Here's how the part is built. I have some questions about the finished solid (model axes, mm). A direction names the side the tool comes from. Give positions to 0.01 mm unless a question says otherwise; leave off trailing zeros. Order: outer loops, then holes, each group sorted by start corner. A loop starts at its lowest first (then second) coordinate and runs counter-clockwise, first axis right, second up.
from build123d import *

# Parameters (mm, degrees)
SKETCH1_R           = 1.5
BOSS_EXTRUDE1_DEPTH = 3
CUT_EXTRUDE1_DEPTH  = 4


with BuildPart() as part:
    # Sketch1 → Boss-Extrude1 (new body)
    with BuildSketch(Plane.XY):
        with BuildLine():
            Line((-36.448598131, -26.168224299), (-36.448598131, -23.168224299))
            Line((-36.448598131, -23.168224299), (-34.837367865, 22.971373688))
            ThreePointArc((-34.837367865, 22.971373688), (-33.618438039, 25.709134902), (-30.839804557, 26.831775701))
            Line((-30.839804557, 26.831775701), (-19.702559656, 26.831775701))
            ThreePointArc((-19.702559656, 26.831775701), (-17.165801235, 25.924485955), (-15.779830266, 23.614204058))
            Line((-15.779830266, 23.614204058), (-6.448598131, -23.168224299))
            Line((-6.448598131, -23.168224299), (-6.448598131, -26.168224299))
            Line((-6.448598131, -26.168224299), (-16.448598131, -26.168224299))
            Line((-16.448598131, -26.168224299), (-16.448598131, -23.168224299))
            Line((-16.448598131, -23.168224299), (-26.448598131, -23.168224299))
            Line((-26.448598131, -23.168224299), (-26.448598131, -26.168224299))
            Line((-26.448598131, -26.168224299), (-36.448598131, -26.168224299))
        make_face()
        with Locations((-21.448598131, 18.831775701)):
            Circle(SKETCH1_R, mode=Mode.SUBTRACT)
        with BuildLine():
            Line((-27.448598131, 4.074261176), (-27.448598131, 0.074261176))
            ThreePointArc((-27.448598131, 0.074261176), (-28.948598131, -1.425738824), (-30.448598131, 0.074261176))
            Line((-30.448598131, 0.074261176), (-30.448598131, 4.074261176))
            ThreePointArc((-30.448598131, 4.074261176), (-28.948598131, 5.574261176), (-27.448598131, 4.074261176))
        make_face(mode=Mode.SUBTRACT)
        with BuildLine():
            Line((-19.448598131, 4.074261176), (-19.448598131, 0.074261176))
            ThreePointArc((-19.448598131, 0.074261176), (-20.948598131, -1.425738824), (-22.448598131, 0.074261176))
            Line((-22.448598131, 0.074261176), (-22.448598131, 4.074261176))
            ThreePointArc((-22.448598131, 4.074261176), (-20.948598131, 5.574261176), (-19.448598131, 4.074261176))
        make_face(mode=Mode.SUBTRACT)
        with BuildLine():
            ThreePointArc((-28.948598131, 18.831775701), (-26.75189899, 13.528474842), (-21.448598131, 11.331775701))
            ThreePointArc((-21.448598131, 11.331775701), (-19.948598131, 12.831775701), (-21.448598131, 14.331775701))
            ThreePointArc((-21.448598131, 14.331775701), (-24.630578646, 15.649795186), (-25.948598131, 18.831775701))
            ThreePointArc((-25.948598131, 18.831775701), (-27.448598131, 20.331775701), (-28.948598131, 18.831775701))
        make_face(mode=Mode.SUBTRACT)
    extrude(amount=BOSS_EXTRUDE1_DEPTH)

    # Sketch2 → Cut-Extrude1 (cut, through all)
    with BuildSketch(Plane.XY.offset(3)):
        Polygon((-34.343835822, -26.168224299), (-34.343835822, -20.168224299), (-36.343835822, -20.168224299), (-36.448598131, -23.168224299), (-36.448598131, -26.168224299), align=None)
    extrude(amount=-CUT_EXTRUDE1_DEPTH, mode=Mode.SUBTRACT)


solid = part.part
Q1. If we section it at C-C on x = -23.75: List the corners of the cut face in (y, z) for me, plus the area to 3 significant figures.
Filled sheet:
outline: (-23.17, 0) - (11.69, 0) - (11.69, 3) - (-23.17, 3) - close; (14.96, 0) - (26.83, 0) - (26.83, 3) - (14.96, 3) - close
area: 140 mm2
Q2. If we section it at B-B on y = 18: List the corners of the cut face in (x, z) for me, plus the area to 3 significant figures.
Filled sheet:
outline: (-35.01, 0) - (-28.9, 0) - (-28.9, 3) - (-35.01, 3) - close; (-25.87, 0) - (-22.7, 0) - (-22.7, 3) - (-25.87, 3) - close; (-20.2, 0) - (-14.66, 0) - (-14.66, 3) - (-20.2, 3) - close
area: 44.5 mm2
Q3. Thinking about a two-plate mould opening in X: for faces 5 (the face through (-25, 1, 3)), 6 (the face through (-17.2, 25.95, 1.48)), 7 (the face through (-28.982, 5.574, 1.479)), which applies, released by +X, released by -X, zero draft, split by the parting line, or undercut?
Filled sheet:
face 5: zero draft
face 6: released by +X
face 7: undercut
Q4. I need wall thicknesses on L1, parallel to Y at x = -29, z = 1.85; L2, parallel to X at y = 4, z = 0.75; L3, parallel to Y at x = -21.5, z = 2.8. Which ranges of each line are inside material? Lowest first, please.
Filled sheet:
L1: y = -26.17 to -1.42, 5.57 to 26.83
L2: x = -35.5 to -30.45, -27.45 to -22.45, -19.45 to -11.87
L3: y = -23.17 to -1.32, 5.47 to 11.33, 14.33 to 17.33, 20.33 to 26.83
Q5. If we section it at D-D on y = 5: List the corners of the cut face in (x, z) for me.
Filled sheet:
outline: (-35.46, 0) - (-30.13, 0) - (-30.13, 3) - (-35.46, 3) - close; (-27.77, 0) - (-22.13, 0) - (-22.13, 3) - (-27.77, 3) - close; (-19.77, 0) - (-12.07, 0) - (-12.07, 3) - (-19.77, 3) - close
Q6. If we section it at A-A on z = 2.15: List the corners of the cut face in (x, y) for me.
Filled sheet:
outline: (-36.34, -20.17) - (-34.34, -20.17) - (-34.34, -26.17) - (-26.45, -26.17) - (-26.45, -23.17) - (-16.45, -23.17) - (-16.45, -26.17) - (-6.45, -26.17) - (-6.45, -23.17) - (-15.78, 23.61) arc R4 ccw to (-19.7, 26.83) - (-30.84, 26.83) arc R4 ccw to (-34.84, 22.97) - close; hole (-30.45, 0.07) arc R1.5 ccw to (-27.45, 0.07) - (-27.45, 4.07) arc R1.5 ccw to (-30.45, 4.07) - close; hole (-28.95, 18.83) arc R7.5 ccw to (-21.45, 11.33) arc R1.5 ccw to (-21.45, 14.33) arc R4.5 cw to (-25.95, 18.83) arc R1.5 ccw to start; hole circle Ø3 at (-21.45, 18.83); hole (-22.45, 0.07) arc R1.5 ccw to (-19.45, 0.07) - (-19.45, 4.07) arc R1.5 ccw to (-22.45, 4.07) - close
Q7. I'm going to push flat-ended pins straight in: P1, Ø1, axis at y = -2.5, z = 2.5, coming from the -X side; P2, Ø0.9, axis at y = 1.5, z = 2, coming from the -X side; P3, Ø1.6, axis at x = -35.5, z = 2, coming from the -Y side. Where does each tip first touch, or does it pass through?
Filled sheet:
P1: stops at x = -35.74
P2: stops at x = -35.6
P3: stops at y = -20.17
Q8. For faces 1 (the face through (-11.18, 0.55, 1.48)), 2 (the face through (-26.449, -25, 1)), 3 (the face through (-24.6, 15.62, 1.48)), 4 (the face through (-34.344, -23, 2)), which set-ups out of +Z, -Z, +X, -X, +Y, -Y let a thin tool reach every point of the face, with its end or its side?
Filled sheet:
face 1: +Z, -Z, +X, +Y
face 2: +Z, -Z, -Y
face 3: +Z, -Z
face 4: +Z, -Z, -X, -Y
